Check sheet for the modelled part. Datum: model origin and axes. Units: mm. Face numbers are marked on the shaded views. A direction names the side the tool comes from. Give positions to 0.01 mm unless a question says otherwise; leave off trailing zeros. Loops run counter-clockwise (first coordinate to the right, second up) from the corner with the lowest first, then second, coordinate; pieces in that order, holes last. Notation, with made-up numbers: (-3, 70.5) - (34, 70.5) arc R6 cw to (34, 75.5) - close; hole circle Ø4 at (26.25, 14.5). An arc over 180 degrees is marked (long way). Use one line per item in the form item = value.
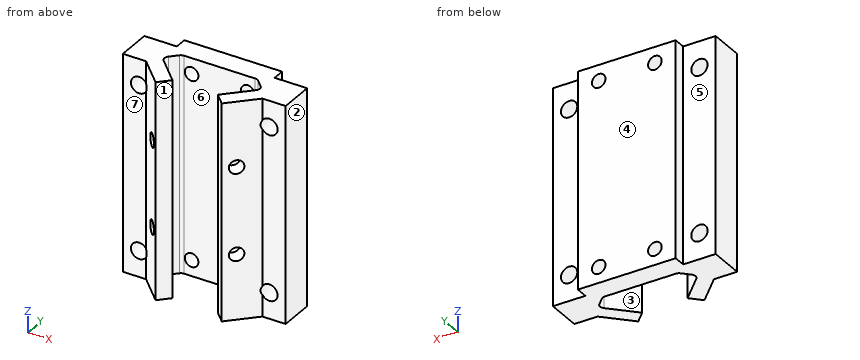
Autodesk Inventor part; units mm, degrees
ref_plane "Carriage Mid Plane" through (0, 15.4627, -63.5) normal (-1, 0, 0) x (0, 0, 1)
ref_plane "Work Plane3" through (0, 0, 48.26) normal (0, 0, 1) x (1, 0, 0)
ref_plane "Work Plane4" through (0, 15.4627, 63.5) normal (-1, 0, 0) x (0, 0, 1)
sketch "Sketch1" plane through (0, 0, 0) normal (0, 0, 1) x (1, 0, 0)
  line L0 (0, 17.9605) -> (17.9605, 0) construction
  line L1 (17.9605, 0) -> (0, -17.9605) construction
  line L2 (0, -17.9605) -> (-17.9605, 0) construction
  line L3 (-17.9605, 0) -> (0, 17.9605) construction
  line L4 (0, 17.9605) -> (0, -17.9605) construction
  line L5 (17.9605, 0) -> (-17.9605, 0) construction
  line L6 (0, -37.7234) -> (0, 100.617)
  line L7 (-27.2882, 23.4644) -> (-11.7319, 7.908) construction
  line L8 (-11.7319, 7.908) -> (-6.7821, 12.8578) construction
  line L9 (-6.7821, 12.8578) -> (-22.3385, 28.4141) construction
  line L10 (-27.2882, 23.4644) -> (-22.3385, 28.4141) construction
  line L11 (27.2882, 23.4644) -> (11.7319, 7.908) construction
  line L12 (11.7319, 7.908) -> (6.7821, 12.8578) construction
  line L13 (6.7821, 12.8578) -> (22.3385, 28.4141) construction
  line L14 (27.2882, 23.4644) -> (22.3385, 28.4141) construction
  line L15 (-13.3307, 6.837) -> (-29.3711, 22.8773)
  line L16 (-29.3711, 22.8773) -> (-22.2034, 30.045)
  line L17 (-22.2034, 30.045) -> (0, 30.045)
  line L18 (-47.8625, 35.7423) -> (-28.7516, 35.7423)
  line L19 (-28.7516, 35.7423) -> (-28.7516, 42.812)
  line L20 (-28.7516, 42.812) -> (0, 42.812)
  line L21 (-47.8625, 15.4627) -> (-47.8625, 35.7423)
  line L22 (-47.8625, 15.4627) -> (-34.2195, 15.4627)
  line L23 (-34.2195, 15.4627) -> (-19.4622, 0.7055)
  line L24 (-19.4622, 0.7055) -> (-13.3307, 6.837)
  line L25 (13.3307, 6.837) -> (29.3711, 22.8773)
  line L26 (29.3711, 22.8773) -> (22.2034, 30.045)
  line L27 (22.2034, 30.045) -> (0, 30.045)
  line L28 (47.8625, 35.7423) -> (28.7516, 35.7423)
  line L29 (28.7516, 35.7423) -> (28.7516, 42.812)
  line L30 (28.7516, 42.812) -> (0, 42.812)
  line L31 (47.8625, 15.4627) -> (47.8625, 35.7423)
  line L32 (47.8625, 15.4627) -> (34.2195, 15.4627)
  line L33 (34.2195, 15.4627) -> (19.4622, 0.7055)
  line L34 (19.4622, 0.7055) -> (13.3307, 6.837)
  line L35 (-9.1166, 42.812) -> (-9.1166, 58.2918)
  line L36 (-9.1166, 58.2918) -> (0, 58.2918)
  point P0 (0, 0)
  point P1 (0, 0)
  point P2 (0, 0)
  point P3 (0, 0)
  dimension "d2" = 25.4
  dimension "d3" = 25.4
  dimension "d6" = 22
  dimension "d14" = 7
extrude "Carriage Frame" add sketch "Sketch1" along normal mid plane 127 contours L17 L16 L15 L24 L23 L22 L21 L18 L19 L20 L6 | L6 L30 L29 L28 L31 L32 L33 L34 L25 L26 L27
fillet "Fillet1" radius 3.175 4 edges at (-29.3711, 22.8773, 0) (-22.2034, 30.045, 0) (22.2034, 30.045, 0) (29.3711, 22.8773, 0)
sketch "Sketch7" plane through (-47.8625, 35.7423, -63.5) normal (0, 1, 0) x (1, 0, 0)
  line L0 (19.1109, 0) -> (76.6141, 0)
  line L1 (19.1109, 0) -> (19.1109, -127)
  line L2 (76.6141, -127) -> (19.1109, -127)
  line L3 (76.6141, 0) -> (76.6141, -127)
  line L4 (0, 0) -> (19.1109, 0)
  line L5 (0, 0) -> (0, -127)
  line L6 (19.1109, -127) -> (0, -127)
  line L7 (19.1109, 0) -> (19.1109, -127)
  line L8 (76.6141, 0) -> (95.725, 0)
  line L9 (76.6141, 0) -> (76.6141, -127)
  line L10 (95.725, -127) -> (76.6141, -127)
  line L11 (95.725, 0) -> (95.725, -127)
  line L12 (19.1109, -63.5) -> (76.6141, -63.5) construction
  line L13 (47.8625, -63.5) -> (47.8625, -63.5) construction
  line L14 (16.8262, -19.4378) -> (9.5554, -23.6355)
  line L15 (9.5554, -23.6355) -> (2.2847, -19.4378)
  line L16 (2.2847, -19.4378) -> (2.2847, -11.0422)
  line L17 (2.2847, -11.0422) -> (9.5554, -6.8445)
  line L18 (9.5554, -6.8445) -> (16.8262, -11.0422)
  line L19 (16.8262, -11.0422) -> (16.8262, -19.4378)
  line L20 (78.8988, -19.4378) -> (86.1695, -23.6355)
  line L21 (86.1695, -23.6355) -> (93.4403, -19.4378)
  line L22 (93.4403, -19.4378) -> (93.4403, -11.0422)
  line L23 (93.4403, -11.0422) -> (86.1695, -6.8445)
  line L24 (86.1695, -6.8445) -> (78.8988, -11.0422)
  line L25 (78.8988, -11.0422) -> (78.8988, -19.4378)
  line L26 (16.8262, -107.5622) -> (9.5554, -103.3645)
  line L27 (9.5554, -103.3645) -> (2.2847, -107.5622)
  line L28 (2.2847, -107.5622) -> (2.2847, -115.9578)
  line L29 (2.2847, -115.9578) -> (9.5554, -120.1555)
  line L30 (9.5554, -120.1555) -> (16.8262, -115.9578)
  line L31 (16.8262, -115.9578) -> (16.8262, -107.5622)
  line L32 (78.8988, -115.9578) -> (78.8988, -107.5622)
  line L33 (86.1695, -120.1555) -> (78.8988, -115.9578)
  line L34 (78.8988, -107.5622) -> (86.1695, -103.3645)
  line L35 (93.4403, -115.9578) -> (86.1695, -120.1555)
  line L36 (93.4403, -107.5622) -> (93.4403, -115.9578)
  line L37 (86.1695, -103.3645) -> (93.4403, -107.5622)
  circle A0 centre (9.5554, -15.24) radius 4.8006
  circle A1 centre (86.1695, -15.24) radius 4.8006
  circle A2 centre (9.5554, -111.76) radius 4.8006
  circle A3 centre (86.1695, -111.76) radius 4.8006
  point P0 (9.5554, 0)
  dimension "d61" = 15.24
  dimension "d78" = 14.5415
  dimension "d79" = 9.6012
extrude "Carriage Screw" cut sketch "Sketch7" against normal through all contours A0 | A1 | A2 | A3
sketch "Ball Bearings" plane through (-13.3307, 6.837, -63.5) normal (0.7071, 0.7071, 0) x (-0.7071, 0.7071, 0)
  line L0 (19.5095, 127) -> (19.5095, 0)
  line L1 (0, 127) -> (19.5095, 127)
  line L2 (0, 0) -> (0, 127)
  line L3 (19.5095, 0) -> (0, 0)
  circle A0 centre (7.62, 88.9) radius 4
  line L4 (19.5095, 63.5) -> (0, 63.5) construction
  circle A1 centre (7.62, 38.1) radius 4
  point P0 (-14.2607, 63.5)
  dimension "d94" = 8
  dimension "d106" = 25.4
  dimension "d107" = 7.62
ref_plane "Carriage Mid Plane" through (0, 15.4627, -63.5) normal (-1, 0, 0) x (0, 0, 1)
extrude "Ball Bearing Hole" cut sketch "Ball Bearings" against normal up to surface (8.6713 mm away) contours A0 | A1
mirror "Mirror4" about plane through (0, 15.4627, -63.5) normal (-1, 0, 0) of "Ball Bearing Hole"
sketch "Sketch23" plane through (-28.7516, 42.812, 63.5) normal (0, 1, 0) x (1, 0, 0)
  circle A0 centre (12.2416, 117.6989) radius 4.0005
  line L0 (28.7516, 152.4) -> (28.7516, -25.4)
  circle A1 centre (45.2616, 117.6989) radius 4.0005
  line L1 (-38.2559, 63.5) -> (95.7591, 63.5)
  circle A2 centre (12.2416, 9.3011) radius 4.0005
  circle A3 centre (45.2616, 9.3011) radius 4.0005
  point P0 (28.7516, 63.5)
  dimension "d141" = 8.001
  dimension "d144" = 33.02
extrude "Extrusion20" cut sketch "Sketch23" against normal blind 16.6853
sketch "Sketch19" plane through (0, 0, 63.5) normal (0, 0, 1) x (1, 0, 0)
  line L0 (-47.8625, 15.4627) -> (-34.2195, 15.4627)
  line L1 (-34.2195, 15.4627) -> (-19.4622, 0.7055)
  line L2 (-19.4622, 0.7055) -> (-13.3307, 6.837)
  line L3 (-13.3307, 6.837) -> (-27.126, 20.6323)
  arc A0 (-27.126, 25.1224) -> (-27.126, 20.6323) centre (-24.8809, 22.8773) ccw
  line L4 (-27.126, 25.1224) -> (-23.1333, 29.1151)
  arc A1 (-20.8883, 30.045) -> (-23.1333, 29.1151) centre (-20.8883, 26.87) ccw
  line L5 (-20.8883, 30.045) -> (20.8883, 30.045)
  arc A2 (23.1333, 29.1151) -> (20.8883, 30.045) centre (20.8883, 26.87) ccw
  line L6 (23.1333, 29.1151) -> (27.126, 25.1224)
  arc A3 (27.126, 20.6323) -> (27.126, 25.1224) centre (24.8809, 22.8773) ccw
  line L7 (27.126, 20.6323) -> (13.3307, 6.837)
  line L8 (13.3307, 6.837) -> (19.4622, 0.7055)
  line L9 (19.4622, 0.7055) -> (34.2195, 15.4627)
  line L10 (34.2195, 15.4627) -> (47.8625, 15.4627)
  line L11 (47.8625, 15.4627) -> (47.8625, 35.7423)
  line L12 (47.8625, 35.7423) -> (28.7516, 35.7423)
  line L13 (28.7516, 35.7423) -> (28.7516, 42.812)
  line L14 (28.7516, 42.812) -> (-28.7516, 42.812)
  line L15 (-28.7516, 42.812) -> (-28.7516, 35.7423)
  line L16 (-28.7516, 35.7423) -> (-47.8625, 35.7423)
  line L17 (-47.8625, 35.7423) -> (-47.8625, 15.4627)
  line L18 (-28.7516, 35.7423) -> (28.7516, 35.7423)
  point P0 (0, 0)
sketch "Sketch20" plane through (0, 0, 0) normal (0, 0, 1) x (1, 0, 0)
  line L0 (-47.8625, 35.7423) -> (47.8625, 35.7423)
  line L1 (47.8625, 35.7423) -> (47.8625, 15.4627)
  line L2 (47.8625, 15.4627) -> (34.2195, 15.4627)
  line L3 (34.2195, 15.4627) -> (19.4622, 0.7055)
  line L4 (19.4622, 0.7055) -> (13.3307, 6.837)
  line L5 (13.3307, 6.837) -> (27.126, 20.6323)
  arc A0 (27.126, 20.6323) -> (27.126, 25.1224) centre (24.8809, 22.8773) ccw
  line L6 (27.126, 25.1224) -> (23.1333, 29.1151)
  arc A1 (23.1333, 29.1151) -> (20.8883, 30.045) centre (20.8883, 26.87) ccw
  line L7 (20.8883, 30.045) -> (-20.8883, 30.045)
  arc A2 (-20.8883, 30.045) -> (-23.1333, 29.1151) centre (-20.8883, 26.87) ccw
  line L8 (-23.1333, 29.1151) -> (-27.126, 25.1224)
  arc A3 (-27.126, 25.1224) -> (-27.126, 20.6323) centre (-24.8809, 22.8773) ccw
  line L9 (-27.126, 20.6323) -> (-13.3307, 6.837)
  line L10 (-13.3307, 6.837) -> (-19.4622, 0.7055)
  line L11 (-19.4622, 0.7055) -> (-34.2195, 15.4627)
  line L12 (-34.2195, 15.4627) -> (-47.8625, 15.4627)
  line L13 (-47.8625, 15.4627) -> (-47.8625, 35.7423)
  line L14 (0, -16.1708) -> (0, 97.0249)
  line L15 (-12.7, 35.7423) -> (-12.7, 61.1423)
  line L16 (-12.7, 61.1423) -> (0, 61.1423)
  line L17 (12.7, 35.7423) -> (12.7, 61.1423)
  line L18 (12.7, 61.1423) -> (0, 61.1423)
  point P0 (0, 0)
  dimension "d131" = 25.4
  dimension "d132" = 12.7
  dimension "d135" = 14.5542
  dimension "d136" = 9.6012
sketch "Sketch13" plane through (0, 0, 63.5) normal (0, 0, 1) x (1, 0, 0)
  line L0 (47.8625, 35.7423) -> (28.7516, 35.7423)
  line L1 (28.7516, 35.7423) -> (28.7516, 42.812)
  line L2 (28.7516, 42.812) -> (-28.7516, 42.812)
  line L3 (-28.7516, 42.812) -> (-28.7516, 35.7423)
  line L4 (-28.7516, 35.7423) -> (-47.8625, 35.7423)
  line L5 (-47.8625, 35.7423) -> (-47.8625, 15.4627)
  line L6 (-47.8625, 15.4627) -> (-34.2195, 15.4627)
  line L7 (-34.2195, 15.4627) -> (-19.4622, 0.7055)
  line L8 (-19.4622, 0.7055) -> (-13.3307, 6.837)
  line L9 (-13.3307, 6.837) -> (-27.126, 20.6323)
  arc A0 (-27.126, 25.1224) -> (-27.126, 20.6323) centre (-24.8809, 22.8773) ccw
  line L10 (-27.126, 25.1224) -> (-23.1333, 29.1151)
  arc A1 (-20.8883, 30.045) -> (-23.1333, 29.1151) centre (-20.8883, 26.87) ccw
  line L11 (-20.8883, 30.045) -> (20.8883, 30.045)
  arc A2 (23.1333, 29.1151) -> (20.8883, 30.045) centre (20.8883, 26.87) ccw
  line L12 (23.1333, 29.1151) -> (27.126, 25.1224)
  arc A3 (27.126, 20.6323) -> (27.126, 25.1224) centre (24.8809, 22.8773) ccw
  line L13 (27.126, 20.6323) -> (13.3307, 6.837)
  line L14 (13.3307, 6.837) -> (19.4622, 0.7055)
  line L15 (19.4622, 0.7055) -> (34.2195, 15.4627)
  line L16 (34.2195, 15.4627) -> (47.8625, 15.4627)
  line L17 (47.8625, 15.4627) -> (47.8625, 35.7423)
  line L18 (-3.175, 42.812) -> (3.175, 42.812)
  line L19 (3.175, 42.812) -> (3.175, 35.1375)
  line L20 (3.175, 35.1375) -> (-3.175, 35.1375)
  line L21 (-3.175, 35.1375) -> (-3.175, 42.812)
  point P0 (0, 0)
  point P1 (0, 42.812)
  point P2 (0, 42.812)
  dimension "d112" = 6.35
sketch "Sketch15" plane through (0, 0, 48.26) normal (0, 0, 1) x (1, 0, 0)
  line L0 (-3.175, 35.1375) -> (-3.175, 42.812)
  line L1 (-3.175, 42.812) -> (-28.7516, 42.812)
  line L2 (-28.7516, 42.812) -> (-28.7516, 35.7423)
  line L3 (-28.7516, 35.7423) -> (-47.8625, 35.7423)
  line L4 (-47.8625, 35.7423) -> (-47.8625, 15.4627)
  line L5 (-47.8625, 15.4627) -> (-34.2195, 15.4627)
  line L6 (-34.2195, 15.4627) -> (-19.4622, 0.7055)
  line L7 (-19.4622, 0.7055) -> (-13.3307, 6.837)
  line L8 (-13.3307, 6.837) -> (-27.126, 20.6323)
  arc A0 (-27.126, 25.1224) -> (-27.126, 20.6323) centre (-24.8809, 22.8773) ccw
  line L9 (-27.126, 25.1224) -> (-23.1333, 29.1151)
  arc A1 (-20.8883, 30.045) -> (-23.1333, 29.1151) centre (-20.8883, 26.87) ccw
  line L10 (-20.8883, 30.045) -> (20.8883, 30.045)
  arc A2 (23.1333, 29.1151) -> (20.8883, 30.045) centre (20.8883, 26.87) ccw
  line L11 (23.1333, 29.1151) -> (27.126, 25.1224)
  arc A3 (27.126, 20.6323) -> (27.126, 25.1224) centre (24.8809, 22.8773) ccw
  line L12 (27.126, 20.6323) -> (13.3307, 6.837)
  line L13 (13.3307, 6.837) -> (19.4622, 0.7055)
  line L14 (19.4622, 0.7055) -> (34.2195, 15.4627)
  line L15 (34.2195, 15.4627) -> (47.8625, 15.4627)
  line L16 (47.8625, 15.4627) -> (47.8625, 35.7423)
  line L17 (47.8625, 35.7423) -> (28.7516, 35.7423)
  line L18 (28.7516, 35.7423) -> (28.7516, 42.812)
  line L19 (28.7516, 42.812) -> (3.175, 42.812)
  line L20 (3.175, 42.812) -> (3.175, 35.1375)
  line L21 (3.175, 35.1375) -> (-3.175, 35.1375)
  line L22 (-3.175, 42.812) -> (-3.175, 80.5116) construction
  line L23 (-3.175, 80.5116) -> (3.175, 80.5116) construction
  line L24 (3.175, 42.812) -> (3.175, 80.5116) construction
  line L25 (-47.8625, 35.7423) -> (-47.8625, 49.9547)
  line L26 (-47.8625, 49.9547) -> (-17.7931, 49.9547)
  line L27 (-17.7931, 49.9547) -> (-17.7931, 73.4726)
  line L28 (-17.7931, 73.4726) -> (-3.175, 73.4726)
  line L29 (-3.175, 73.4726) -> (-3.175, 42.812)
  line L30 (-28.7516, 42.812) -> (-28.7516, 35.7423)
  point P0 (0, 0)
sketch "Sketch16" plane through (-47.8625, 49.9547, 58.42) normal (0, 1, 0) x (1, 0, 0)
  circle A0 centre (9.5554, 10.16) radius 4.8006
  point P0 (47.8625, 58.42)
sketch "Sketch17" plane through (-17.7931, 49.9547, 58.42) normal (-1, 0, 0) x (0, 0, 1)
  line L0 (-20.32, 0) -> (0, 0)
  line L1 (0, 23.5178) -> (0, 0)
  line L2 (-20.32, 23.5178) -> (0, 23.5178)
  line L3 (-20.32, 0) -> (-20.32, 23.5178)
  circle A0 centre (-10.16, 11.7589) radius 4
  point P0 (-58.42, -49.9547)
  point P1 (-10.16, 23.5178)
  point P2 (0, 11.7589)
  dimension "d122" = 8
equation "\"carriage_length\" = 127"
equation "\"ball_bearing_diam\" = 22"
equation "\"ball_bearing_hole\" = 8"
equation "\"d92\" = 8"
properties part number "universal_carriage" material "ABS Plastic"
Item 1: Gauge pin test, flat ends, axial feed: P1, Ø4, axis at x = 37.5, z = -28.5, coming from the -Y side; P2, Ø6, axis at x = 28, z = -22.5, coming from the -Y side; P3, Ø9.5, axis at x = 37, z = -3.5, coming from the +Y side; P4, Ø8.5, axis at x = -38.31, z = 48.26, coming from the -Y side (3 decimals). Record the tip position at first contact, or that the pin passes through.
Answer block:
P1 = 15.46
P2 = 6.44
P3 = 35.74
P4 = through
Item 2: Mould release check, pull along X, two halves, no side actions. Record for the marked faces 1, 2, 3 and 4: released by +X, released by -X, zero draft, split by the parting line, or undercut.
Answer block:
face_1 = undercut
face_2 = released by +X
face_3 = undercut
face_4 = zero draft
Item 3: Access from +Z, -Z, +X, -X, +Y, -Y to the whole of each face (thin tool, end or side, straight path). Record for the marked faces 5, 6 and 7.
Answer block:
face_5 = +Z, -Z, -X, +Y
face_6 = +Z, -Z
face_7 = +Z, -Z, -X, -Y
Item 4: Section check C-C on y = 40.5. Record the boundary of the cut face in (x, z), then the cut area to 3 significant figures.
Answer block:
outline = (-28.75, -63.5) - (28.75, -63.5) - (28.75, 63.5) - (-28.75, 63.5) - close; hole circle Ø8 at (-16.51, -54.2); hole circle Ø8 at (-16.51, 54.2); hole circle Ø8 at (16.51, -54.2); hole circle Ø8 at (16.51, 54.2)
area = 7,100 mm2
Item 5: Section check A-A on z = 48.26. Give the number of separate pieces and of enclosed holes in the cut face, then the cut area to 3 significant figures.
Answer block:
separate_pieces = 3
enclosed_holes = 0
area = 1,500 mm2
Item 6: Thickness scan on L1, parallel to Z at x = -16.51, y = 38.25; L2, parallel to Z at x = 14, y = 30.5; L3, parallel to Y at x = -7.5, z = 51 (3 decimals). Record the ranges inside material, lowest first.
Answer block:
L1 = -63.5 to -58.2, -50.2 to 50.2, 58.2 to 63.5
L2 = -63.5 to -57.31, -51.08 to 51.08, 57.31 to 63.5
L3 = 30.045 to 42.812
